```python
from build123d import *

# Parameters (mm, degrees)
EXTRUDE_1_DEPTH     = 40
CUT_EXTRUDE_1_REACH = 60.034
SKETCH_2_R          = 2.2
CUT_EXTRUDE_2_REACH = 60.034
SKETCH_3_R          = 1.7


with BuildPart() as part:
    # 草图1 → 凸台-拉伸1 (new body)
    with BuildSketch(Plane.XY):
        Polygon((0, 0), (18, 0), (18, -38), (16, -38), (16, -2), (0, -2), align=None)
    extrude(amount=EXTRUDE_1_DEPTH)

    # 草图2 → 切除-拉伸1 (cut, up to next)
    with BuildSketch(Plane(origin=(0, 0, 0), x_dir=(1, 0, 0), z_dir=(0, 1, 0)), mode=Mode.PRIVATE) as cut_extrude_1_sk1:
        with Locations(Location((6, -28, 0), (0, 0, 270))):
            Circle(SKETCH_2_R)
    cut_extrude_1_tool1 = extrude(cut_extrude_1_sk1.sketch, amount=-CUT_EXTRUDE_1_REACH, mode=Mode.PRIVATE) & part.part
    # 草图2 → 切除-拉伸1 (cut, up to next)
    with BuildSketch(Plane(origin=(0, 0, 0), x_dir=(1, 0, 0), z_dir=(0, 1, 0)), mode=Mode.PRIVATE) as cut_extrude_1_sk2:
        with Locations(Location((6, -12, 0), (0, 0, 270))):
            Circle(SKETCH_2_R)
    cut_extrude_1_tool2 = extrude(cut_extrude_1_sk2.sketch, amount=-CUT_EXTRUDE_1_REACH, mode=Mode.PRIVATE) & part.part
    add(cut_extrude_1_tool1.solids().sort_by_distance((6, 0, 28))[0], mode=Mode.SUBTRACT)
    add(cut_extrude_1_tool2.solids().sort_by_distance((6, 0, 12))[0], mode=Mode.SUBTRACT)

    # 草图3 → 切除-拉伸2 (cut, up to next)
    with BuildSketch(Plane(origin=(18, 0, 0), x_dir=(0, 0, -1), z_dir=(1, 0, 0)), mode=Mode.PRIVATE) as cut_extrude_2_sk1:
        with Locations(Location((-27.5, -15, 0), (0, 0, 90))):
            Circle(SKETCH_3_R)
    cut_extrude_2_tool1 = extrude(cut_extrude_2_sk1.sketch, amount=-CUT_EXTRUDE_2_REACH, mode=Mode.PRIVATE) & part.part
    # 草图3 → 切除-拉伸2 (cut, up to next)
    with BuildSketch(Plane(origin=(18, 0, 0), x_dir=(0, 0, -1), z_dir=(1, 0, 0)), mode=Mode.PRIVATE) as cut_extrude_2_sk2:
        with Locations(Location((-12.5, -15, 0), (0, 0, 90))):
            Circle(SKETCH_3_R)
    cut_extrude_2_tool2 = extrude(cut_extrude_2_sk2.sketch, amount=-CUT_EXTRUDE_2_REACH, mode=Mode.PRIVATE) & part.part
    # 草图3 → 切除-拉伸2 (cut, up to next)
    with BuildSketch(Plane(origin=(18, 0, 0), x_dir=(0, 0, -1), z_dir=(1, 0, 0)), mode=Mode.PRIVATE) as cut_extrude_2_sk3:
        with Locations(Location((-36, -4, 0), (0, 0, 90))):
            Circle(SKETCH_3_R)
    cut_extrude_2_tool3 = extrude(cut_extrude_2_sk3.sketch, amount=-CUT_EXTRUDE_2_REACH, mode=Mode.PRIVATE) & part.part
    # 草图3 → 切除-拉伸2 (cut, up to next)
    with BuildSketch(Plane(origin=(18, 0, 0), x_dir=(0, 0, -1), z_dir=(1, 0, 0)), mode=Mode.PRIVATE) as cut_extrude_2_sk4:
        with Locations(Location((-4, -4, 0), (0, 0, 90))):
            Circle(SKETCH_3_R)
    cut_extrude_2_tool4 = extrude(cut_extrude_2_sk4.sketch, amount=-CUT_EXTRUDE_2_REACH, mode=Mode.PRIVATE) & part.part
    add(cut_extrude_2_tool1.solids().sort_by_distance((18, -15, 27.5))[0], mode=Mode.SUBTRACT)
    add(cut_extrude_2_tool2.solids().sort_by_distance((18, -15, 12.5))[0], mode=Mode.SUBTRACT)
    add(cut_extrude_2_tool3.solids().sort_by_distance((18, -4, 36))[0], mode=Mode.SUBTRACT)
    add(cut_extrude_2_tool4.solids().sort_by_distance((18, -4, 4))[0], mode=Mode.SUBTRACT)


solid = part.part
```
Read the model definition and answer for the solid it produces. Units are mm, in the model's axes. A direction names the side the tool comes from. Coordinates: 2 decimals unless noted, no trailing zeros. Loops run counter-clockwise (first coordinate to the right, second up) from the corner with the lowest first, then second, coordinate; pieces in that order, holes last. Notation, with made-up numbers: (34.25, 9) - (40.25, 9) arc R10 cw to (40.25, 14) - close; hole circle Ø7 at (20, 64.25). An arc over 180 degrees is marked (long way). Answer in a Markdown table with one row per item.
1. Straight lines are drawn through the part: line 1 (Z direction, x = 17.2, y = -4); line 2 (Z direction, x = 16.75, y = -15); line 3 (X direction, y = -2.5, z = 5). For each, find the intervals that lie inside material, in ascending order.
Conclusion:
| item | result |
|---|---|
| line 1 | z = 0 to 2.3, 5.7 to 34.3, 37.7 to 40 |
| line 2 | z = 0 to 10.8, 14.2 to 25.8, 29.2 to 40 |
| line 3 | x = 16 to 18 |
2. Which of the six approach directions +Z, -Z, +X, -X, +Y, -Y give full straight-line access (tool end or side, diameter ignored) to faces 4 (the face through (8, -2, 20)), 5 (the face through (17.014, -14.086, 28.933))?
Conclusion:
| item | result |
|---|---|
| face 4 | +Z, -Z, -X, -Y |
| face 5 | +X, -X |
3. Find section D-D, the plane z = 28. Write down the section's boundary in (x, y), then the cut area to 3 significant figures.
Conclusion:
| item | result |
|---|---|
| outline | (0, -2) - (3.8, -2) - (3.8, 0) - (0, 0) - close; (8.2, -2) - (16, -2) - (16, -13.38) - (18, -13.38) - (18, 0) - (8.2, 0) - close; (16, -38) - (18, -38) - (18, -16.62) - (16, -16.62) - close |
| area | 92.7 mm² |
4. Determine the mould class of faces 1 (the face through (16.4, -14.7, 40)), 2 (the face through (16, -20, 20)), 3 (the face through (17.01, -2.43, 3.35)) for opening direction Z: +Z half, -Z half, draft (parallel to the pull), parting line (faces both ways), or undercut.
Conclusion:
| item | result |
|---|---|
| face 1 | +Z half |
| face 2 | draft |
| face 3 | undercut |
5. Find section C-C, the plane y = -15. Write down the section's boundary in (x, z), then the cut area to 3 significant figures.
Conclusion:
| item | result |
|---|---|
| outline | (16, 0) - (18, 0) - (18, 10.8) - (16, 10.8) - close; (16, 14.2) - (18, 14.2) - (18, 25.8) - (16, 25.8) - close; (16, 29.2) - (18, 29.2) - (18, 40) - (16, 40) - close |
| area | 66.4 mm² |
6. Find section B-B, the plane z = 36. Write down the section's boundary in (x, y).
Conclusion:
| item | result |
|---|---|
| outline | (0, -2) - (16, -2) - (16, -2.3) - (18, -2.3) - (18, 0) - (0, 0) - close; (16, -38) - (18, -38) - (18, -5.7) - (16, -5.7) - close |
7. Given pin 1 (18 mm diameter, centred on y = -12.5, z = 27.5, fed in from -X); pin 2 (1 mm diameter, centred on x = 5, z = 34.5, fed in from -Y); pin 3 (3 mm diameter, centred on y = -4, z = 4, fed in from +X), each flat-ended and moving along its own axis, determine where each tip first touches the part or whether it passes through.
Conclusion:
| item | result |
|---|---|
| pin 1 | stops at x = 16 |
| pin 2 | stops at y = -2 |
| pin 3 | passes through |
8. Find section A-A, the plane x = 6. Write down the section's boundary in (y, z).
Conclusion:
| item | result |
|---|---|
| outline | (-2, 0) - (0, 0) - (0, 9.8) - (-2, 9.8) - close; (-2, 14.2) - (0, 14.2) - (0, 25.8) - (-2, 25.8) - close; (-2, 30.2) - (0, 30.2) - (0, 40) - (-2, 40) - close |
